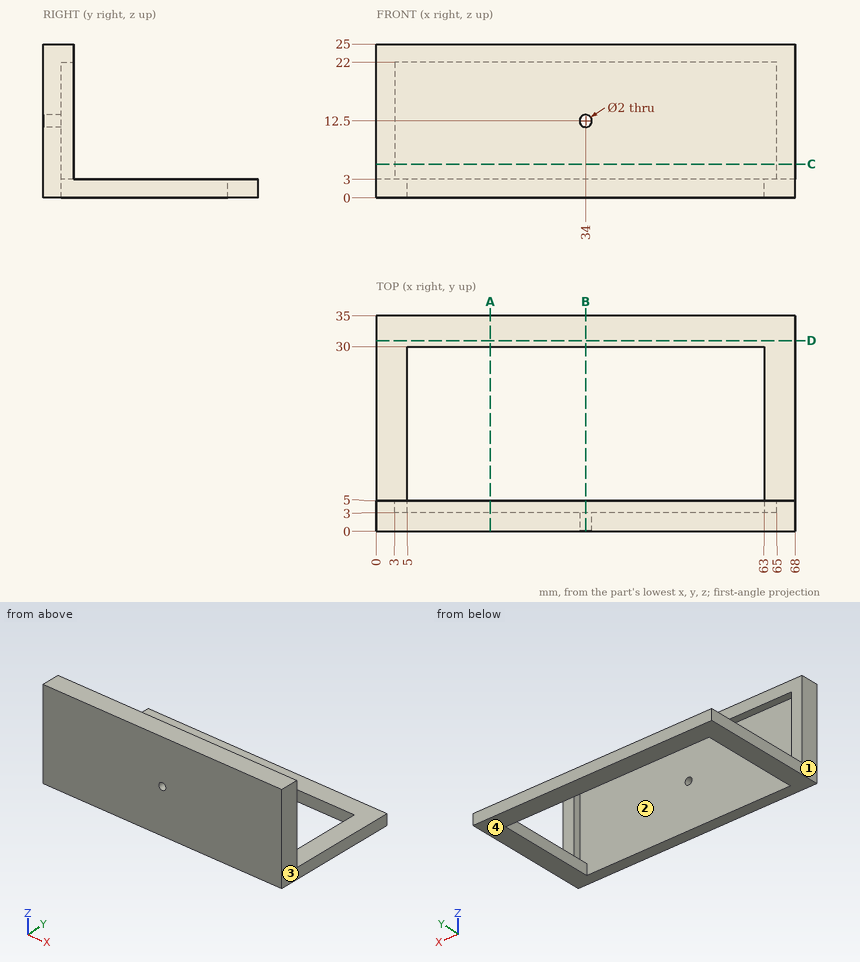
For this review, use the dimensioned drawing (mm, ordinates from the lowest corner) and the shaded views. Coordinates: 2 decimals unless noted, no trailing zeros. Loops run counter-clockwise (first coordinate to the right, second up) from the corner with the lowest first, then second, coordinate; pieces in that order, holes last. Notation, with made-up numbers: M 39,76.25 L 63,76.25 A33 ccw 63,104.25 Z; hole C 34,51.25 d7. An arc over 180 degrees is marked long. Answer as CSV lines item,"result".
Item 1: The part is to be moulded in two halves that separate along X. For the marked faces 1, 2, 3 and 4, say which applies: pulls with the +X half, pulls with the -X half, needs draft (parallel to the pull), parting line crosses it, or undercut.
Answer list:
face 1,"pulls with the -X half"
face 2,"undercut"
face 3,"pulls with the +X half"
face 4,"needs draft"
Item 2: For P1, Ø6.5, axis at x = 27.5, z = 11.5, coming from the +Y side; P2, Ø0.6, axis at x = 35.5, y = 4, coming from the -Z side; P3, Ø10, axis at x = 48, z = 20, coming from the +Y side, all flat-tipped, find the tip position at first contact; note any pin that passes through.
Answer list:
P1,"y = 3"
P2,"z = 22"
P3,"y = 5"
Item 3: Add section C-C on z = 5.5. State the section outline as (x, y) points, plus the area to 3 significant figures.
Answer list:
outline,"M 0,0 L 68,0 L 68,5 L 65,5 L 65,3 L 3,3 L 3,5 L 0,5 Z"
area,"216 mm²"
Item 4: Add section A-A on x = 18.5. State the section outline as (y, z) points.
Answer list:
outline,"M 0,0 L 3,0 L 3,22 L 5,22 L 5,25 L 0,25 Z; M 30,0 L 35,0 L 35,3 L 30,3 Z"
Item 5: Add section D-D on y = 31. State the section outline as (x, z) points.
Answer list:
outline,"M 0,0 L 68,0 L 68,3 L 0,3 Z"
Item 6: Add section B-B on x = 34. State the section outline as (y, z) points, plus the area to 3 significant figures.
Answer list:
outline,"M 0,0 L 3,0 L 3,11.5 L 0,11.5 Z; M 0,13.5 L 3,13.5 L 3,22 L 5,22 L 5,25 L 0,25 Z; M 30,0 L 35,0 L 35,3 L 30,3 Z"
area,"90.0 mm²"
Item 7: For probe 1 along Y at (x, z) = (43, 2.25); probe 2 along Z at (x, y) = (34, 1.75); probe 3 along X at (y, z) = (16, 2), list the stretches that pass through material, from the lowest coordinate up.
Answer list:
probe 1,"0 to 3, 30 to 35"
probe 2,"0 to 11.5, 13.5 to 25"
probe 3,"0 to 5, 63 to 68"
